Read the model definition and answer for the solid it produces. Units are mm, in the model's axes. Round coordinates to 2 decimals unless told otherwise and drop trailing zeros. Write each loop counter-clockwise with the first axis right and the second up, starting at its lowest first coordinate (ties: lowest second). Pieces come first, ordered by that corner, then holes. Notation, with made-up numbers: (71, -14.5) - (120, -14.5) arc R17 cw to (120, -1.5) - close; hole circle Ø11 at (26, 33). An arc over 180 degrees is marked (long way). Use one line per item in the form item = value. Start each with the question number.
1) The part is cut by section C-C, the plane x = 16.51. Count the separate pieces of the cut face and the enclosed holes in it, plus the area to 3 significant figures.
2) The part is cut by section B-B, the plane y = 40. Give the vertices of the cut face in (x, z) (3 decimals), plus the area to 3 significant figures.
3) Each of these flat-tipped pins is pushed along its axis until it touches: pin 1 (1.6 mm diameter, centred on x = 32.5, z = 2.5, fed in from -Y); pin 2 (1 mm diameter, centred on x = 41.5, z = 2, fed in from -Y) (3 decimals); pin 3 (1 mm diameter, centred on y = 9.5, z = 0.5, fed in from +X). Where does it stop, or does it pass through?
4) The part is cut by section A-A, the plane x = 7.5. Give the vertices of the cut face in (y, z) (3 decimals), plus the area to 3 significant figures.
5) Consider line 1 along Y through (x, z) = (16.5, 0.5) (3 decimals); line 2 along X through (y, z) = (23, 0.6); line 3 along Y through (x, z) = (14, 2.35) (3 decimals). Determine where each line is inside the solid, lowest interval first. Write a range as from..to.
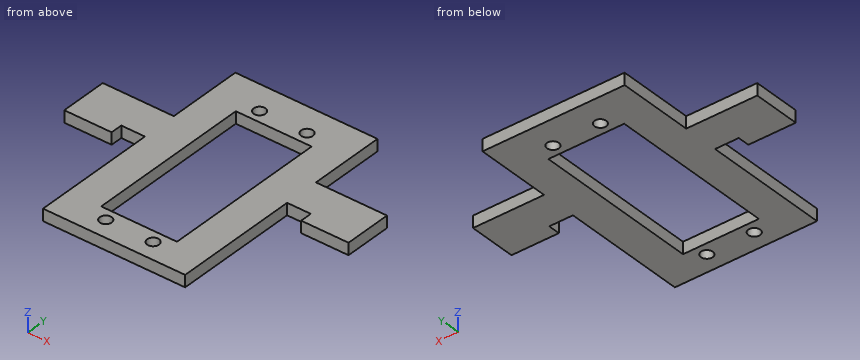
from build123d import *

# Parameters (mm, degrees)
SKETCH1_R           = 1.5875
SKETCH1_W           = 20.32
SKETCH1_H           = 44.45
BOSS_EXTRUDE1_DEPTH = 3.175


with BuildPart() as part:
    # Sketch1 → Boss-Extrude1 (new body)
    with BuildSketch(Plane.XY):
        Polygon((-8.89, 25.4), (-15.24, 25.4), (-15.24, 22.225), (-27.94, 22.225), (-27.94, 34.925), (-8.89, 34.925), (-8.89, 55.245), (29.21, 55.245), (29.21, 34.925), (48.26, 34.925), (48.26, 22.225), (35.56, 22.225), (35.56, 25.4), (29.21, 25.4), (29.21, -8.255), (-8.89, -8.255), align=None)
        with Locations((3.81, 47.625)):
            Circle(SKETCH1_R, mode=Mode.SUBTRACT)
        with Locations((16.51, 47.625)):
            Circle(SKETCH1_R, mode=Mode.SUBTRACT)
        with Locations(Location((16.51, -3.175, 0), (0, 0, 180))):
            Circle(SKETCH1_R, mode=Mode.SUBTRACT)
        with Locations(Location((3.81, -3.175, 0), (0, 0, 180))):
            Circle(SKETCH1_R, mode=Mode.SUBTRACT)
        with Locations((10.16, 22.225)):
            Rectangle(SKETCH1_W, SKETCH1_H, mode=Mode.SUBTRACT)
    extrude(amount=BOSS_EXTRUDE1_DEPTH)


solid = part.part
Geometry results:
q1.separate_pieces = 4
q1.enclosed_holes = 0
q1.area = 40.3 mm2
q2.outline = (-8.89, 0) - (0, 0) - (0, 3.175) - (-8.89, 3.175) - close; (20.32, 0) - (29.21, 0) - (29.21, 3.175) - (20.32, 3.175) - close
q2.area = 56.5 mm2
q3.pin_1 = 25.4
q3.pin_2 = 22.225
q3.pin_3 = 29.21
q4.outline = (-8.255, 0) - (0, 0) - (0, 3.175) - (-8.255, 3.175) - close; (44.45, 0) - (55.245, 0) - (55.245, 3.175) - (44.45, 3.175) - close
q4.area = 60.5 mm2
q5.line_1 = -8.255..-4.762, -1.588..0, 44.45..46.038, 49.212..55.245
q5.line_2 = -27.94..-15.24, -8.89..0, 20.32..29.21, 35.56..48.26
q5.line_3 = -8.255..0, 44.45..55.245
